The listing builds one solid part. Answer for the finished solid, in the listing's coordinates (mm). Coordinates: 2 decimals unless noted, no trailing zeros. Order: outer loops, then holes, each group sorted by start corner. A loop starts at its lowest first (then second) coordinate and runs counter-clockwise, first axis right, second up. Notation, with made-up numbers: (47.25, 36) - (75.25, 36) arc R13 ccw to (75.25, 57) - close; hole circle Ø3 at (52.5, -1.5). An arc over 180 degrees is marked (long way). One line per item, written item: value. Start each with the question number.
```python
from build123d import *

# Parameters (mm, degrees)
SKETCH002_W  = 170.028106
SKETCH002_H  = 154.781021
PAD002_DEPTH = 30
SKETCH001_W  = 178.926751
SKETCH001_H  = 164.552085
PAD_DEPTH    = 25
PAD001_DEPTH = 10


with BuildPart() as pad002:
    # Sketch002 → Pad002 (new body)
    with BuildSketch(Plane.YZ):
        with Locations((0.462036, 0.231018)):
            Rectangle(SKETCH002_W, SKETCH002_H)
    extrude(amount=PAD002_DEPTH)


with BuildPart() as pad:
    # Sketch001 → Pad (new body)
    with BuildSketch(Plane.YZ):
        with Locations((1.16814, -0.450252)):
            Rectangle(SKETCH001_W, SKETCH001_H)
    extrude(amount=PAD_DEPTH)


with BuildPart() as common:
    # Sketch → Pad001 (new body)
    with BuildSketch(Plane.XY):
        Polygon((0, 25), (0, 75), (50, 25), align=None)
    extrude(amount=PAD001_DEPTH)

    # Cut: cut Pad
    add(pad.part, mode=Mode.SUBTRACT)

    # Common: intersect Pad002
    add(pad002.part, mode=Mode.INTERSECT)


solid = common.part
```
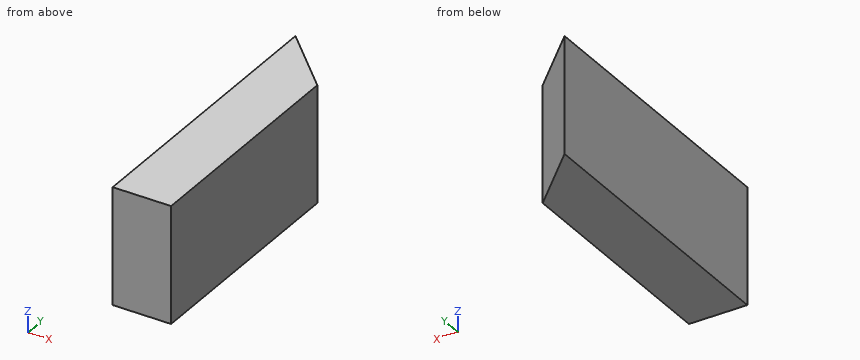
(1) Consider probe 1 along Y at (x, z) = (27.6, 5); probe 2 along Y at (x, z) = (28.8, 6.5); probe 3 along X at (y, z) = (47.5, 8.25). Determine where each line is inside the solid, lowest interval first.
(2) A flat-ended cylindrical pin translates along its axis: pin 1 Ø3 at (x, z) = (28, 4) entering from +Y. Find the tip coordinate at first contact, or state that the pin passes through.
(3) The part is cut by section B-B on y = 46. Determine the outline of the cut face in (x, z).
(4) The part is cut by section A-A on x = 29.65. Determine the outline of the cut face in (y, z).
Completed:
1. probe 1: y = 25 to 47.4
1. probe 2: y = 25 to 46.2
1. probe 3: x = 25 to 27.5
2. pin 1: stops at y = 48.5
3. outline: (25, 0) - (29, 0) - (29, 10) - (25, 10) - close
4. outline: (25, 0) - (45.35, 0) - (45.35, 10) - (25, 10) - close
